Here's the drawing with two shaded views (mm, measured from the low corner). I have some questions. A direction names the side the tool comes from. Round coordinates to 2 decimals unless told otherwise and drop trailing zeros. Order: outer loops, then holes, each group sorted by start corner. A loop starts at its lowest first (then second) coordinate and runs counter-clockwise, first axis right, second up.
Q1. If we section it at D-D (z = 14.25): Please give me the cut outline in (x, y), plus the area to 3 significant figures.
Q2. If we section it at A-A (z = 7.5): Please give me the cut outline in (x, y), plus the area to 3 significant figures.
Q3. If we section it at B-B (x = 5.75): Please give me the cut outline in (y, z).
Q4. Will these pins go through, and if not, where does the flat tip stop? P1, Ø3, axis at y = 27.5, z = 3.5, coming from the -X side; P2, Ø7.5, axis at y = 20, z = 10.5, coming from the +X side; P3, Ø6.5, axis at x = 5.75, z = 7.5, coming from the +Y side.
Q5. If I drill on line 1 (X direction, y = 23, z = 2.25); line 2 (Y direction, x = 25.5, z = 5); line 3 (Y direction, x = 3, z = 11), over which ranges is the centre line in solid material (lowest first)?
Q6. We'd pull the mould along Y, two halves only. Please class the marked faces 1, 2 and 3: pulls with the +Y half, pulls with the -Y half, needs draft (parallel to the pull), parting line crosses it, or undercut.
Q7. If we section it at C-C (y = 23.35): Please give me the cut outline in (x, z).
Q8. For the marked faces 4, 5, 6 and 7, which set-ups out of +Z, -Z, +X, -X, +Y, -Y let a thin tool reach every point of the face, with its end or its side?
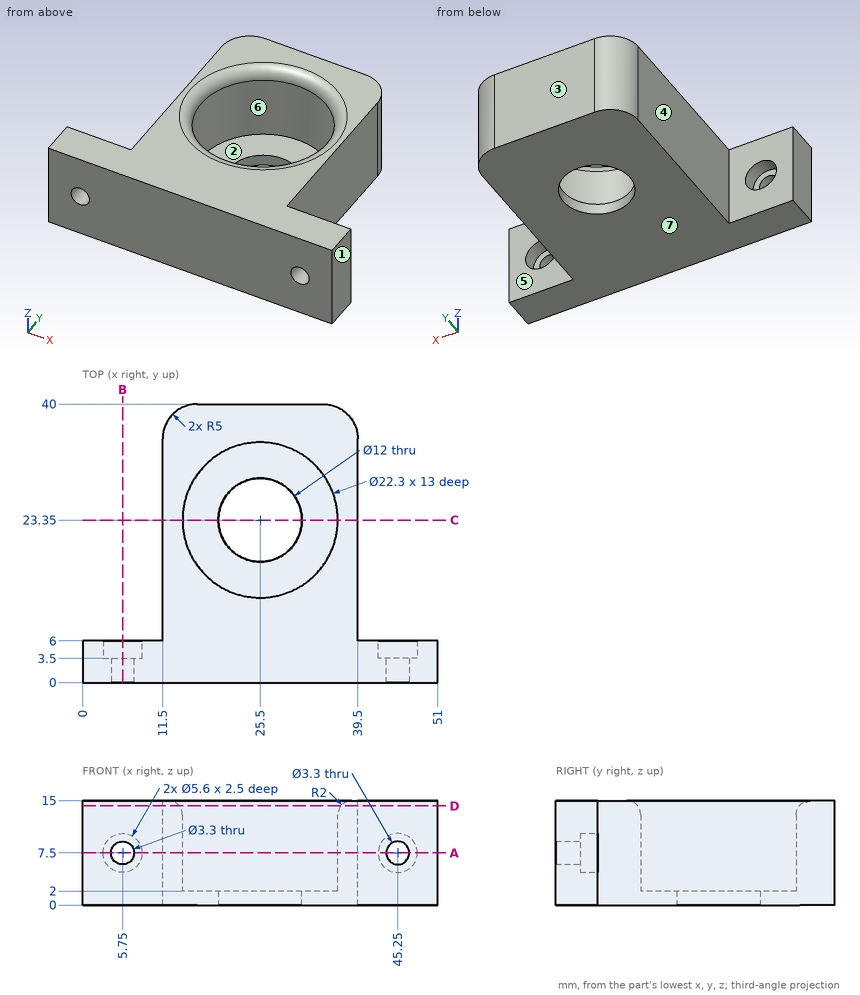
Solution:
1. outline: (0, 0) - (51, 0) - (51, 6) - (39.5, 6) - (39.5, 35) arc R5 ccw to (34.5, 40) - (16.5, 40) arc R5 ccw to (11.5, 35) - (11.5, 6) - (0, 6) - close; hole circle Ø23.18 at (25.5, 23.35)
1. area: 825 mm2
2. outline: (0, 0) - (4.1, 0) - (4.1, 3.5) - (2.95, 3.5) - (2.95, 6) - (0, 6) - close; (7.4, 0) - (43.6, 0) - (43.6, 3.5) - (42.45, 3.5) - (42.45, 6) - (39.5, 6) - (39.5, 35) arc R5 ccw to (34.5, 40) - (16.5, 40) arc R5 ccw to (11.5, 35) - (11.5, 6) - (8.55, 6) - (8.55, 3.5) - (7.4, 3.5) - close; (46.9, 0) - (51, 0) - (51, 6) - (48.05, 6) - (48.05, 3.5) - (46.9, 3.5) - close; hole circle Ø22.3 at (25.5, 23.35)
2. area: 806 mm2
3. outline: (0, 0) - (6, 0) - (6, 4.7) - (3.5, 4.7) - (3.5, 5.85) - (0, 5.85) - close; (0, 9.15) - (3.5, 9.15) - (3.5, 10.3) - (6, 10.3) - (6, 15) - (0, 15) - close
4. P1: stops at x = 11.5
4. P2: stops at x = 39.5
4. P3: stops at y = 6
5. line 1: x = 11.5 to 14.36, 36.64 to 39.5
5. line 2: y = 0 to 12.2, 34.5 to 40
5. line 3: y = 0 to 6
6. face 1: needs draft
6. face 2: undercut
6. face 3: pulls with the +Y half
7. outline: (11.5, 0) - (19.5, 0) - (19.5, 2) - (14.35, 2) - (14.35, 13) arc R2 ccw to (12.35, 15) - (11.5, 15) - close; (31.5, 0) - (39.5, 0) - (39.5, 15) - (38.65, 15) arc R2 ccw to (36.65, 13) - (36.65, 2) - (31.5, 2) - close
8. face 4: +Z, -Z, -X, +Y
8. face 5: +Z, -Z, +X, +Y
8. face 6: +Z
8. face 7: -Z, +X, -X, +Y, -Y
